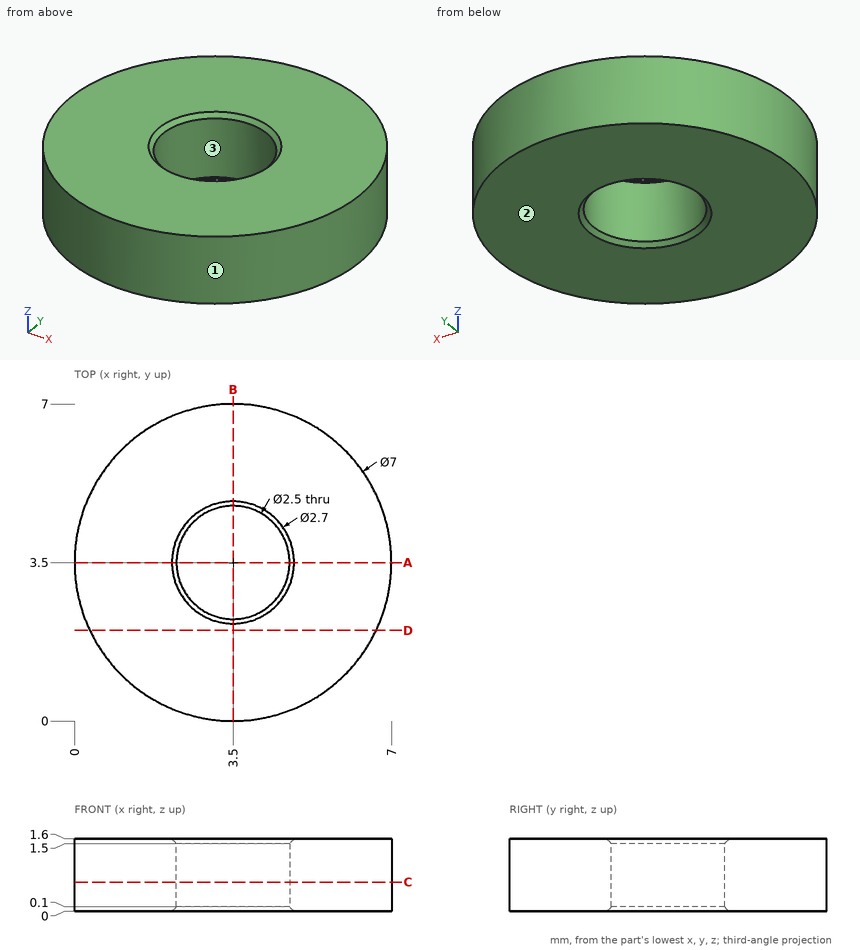
Design review of the part shown in the three views and the two pictorial views. Dimensions are in mm from the part's minimum x, y and z. Round coordinates to 2 decimals unless told otherwise and drop trailing zeros. Order: outer loops, then holes, each group sorted by start corner. A loop starts at its lowest first (then second) coordinate and runs counter-clockwise, first axis right, second up.
Q1. Wall thickness on line 1 (Y direction, x = 3.5, z = 0.65); line 2 (Y direction, x = 4.5, z = 1.25); line 3 (X direction, y = 5.5, z = 0.2): over which ranges is each line inside the solid? List them lowest first.
Findings below:
line 1: y = 0 to 2.25, 4.75 to 7
line 2: y = 0.15 to 2.75, 4.25 to 6.85
line 3: x = 0.63 to 6.37
Q2. Mouldability with a two-part tool opening along Y and no side actions: class the marked faces 1, 2 and 3 as pulls with the +Y half, pulls with the -Y half, needs draft (parallel to the pull), parting line crosses it, or undercut.
Findings below:
face 1: parting line crosses it
face 2: needs draft
face 3: undercut
Q3. We need section A-A, the plane y = 3.5. Give the boundary of the cut face in (x, z).
Findings below:
outline: (0, 0) - (2.15, 0) - (2.25, 0.1) - (2.25, 1.5) - (2.15, 1.6) - (0, 1.6) - close; (4.75, 0.1) - (4.85, 0) - (7, 0) - (7, 1.6) - (4.85, 1.6) - (4.75, 1.5) - close
Q4. Insertion check: P1, Ø3, axis at x = 3.5, y = 3.5, coming from the +Z side. The pin has a flat end and moves straight along its axis. Give the tip position at first contact, or say it passes through.
Findings below:
P1: stops at z = 1.6
Q5. We need section C-C, the plane z = 0.65. Give the boundary of the cut face in (x, y), plus the area to 3 significant figures.
Findings below:
outline: circle Ø7 at (3.5, 3.5); hole circle Ø2.5 at (3.5, 3.5)
area: 33.6 mm2
Q6. We need section D-D, the plane y = 2. Give the boundary of the cut face in (x, z), plus the area to 3 significant figures.
Findings below:
outline: (0.34, 0) - (6.66, 0) - (6.66, 1.6) - (0.34, 1.6) - close
area: 10.1 mm2
